Geometry: final body of the model. Coordinates: model frame, mm. A direction names the side the tool comes from. Give positions to 0.01 mm unless a question says otherwise; leave off trailing zeros. Loops run counter-clockwise (first coordinate to the right, second up) from the corner with the lowest first, then second, coordinate; pieces in that order, holes last.
from build123d import *

# Parameters (mm, degrees)
ESQUISSE1_W             = 80
ESQUISSE1_H             = 35
BOSS_EXTRU_1_DEPTH      = 5
ESQUISSE2_R             = 1.5
ESQUISSE2_R_2           = 1.3
ENL_V_MAT_EXTRU_1_DEPTH = 88.464278423
ESQUISSE4_R             = 2.5
ENL_V_MAT_EXTRU_2_DEPTH = 3
CONG_1_R                = 3


with BuildPart() as part:
    # Esquisse1 → Boss.-Extru.1 (new body)
    with BuildSketch(Plane(origin=(0, 0, 0), x_dir=(1, 0, 0), z_dir=(0, 1, 0))):
        with Locations((40, 17.5)):
            Rectangle(ESQUISSE1_W, ESQUISSE1_H)
    extrude(amount=BOSS_EXTRU_1_DEPTH)

    # Esquisse2 → Enlèv. mat.-Extru.1 (cut, through all)
    with BuildSketch(Plane(origin=(0, 5, 0), x_dir=(1, 0, 0), z_dir=(0, 1, 0))):
        with Locations(Location((5.5, 30, 0), (0, 0, 270))):
            Circle(ESQUISSE2_R)
        with Locations(Location((74.5, 30, 0), (0, 0, 270))):
            Circle(ESQUISSE2_R)
        with Locations(Location((29.270489512, 17.5, 0), (0, 0, 270))):
            Circle(ESQUISSE2_R_2)
        with Locations(Location((54.270489512, 17.5, 0), (0, 0, 270))):
            Circle(ESQUISSE2_R_2)
        with Locations(Location((74.5, 5, 0), (0, 0, 270))):
            Circle(ESQUISSE2_R)
        with Locations(Location((5.5, 5, 0), (0, 0, 270))):
            Circle(ESQUISSE2_R)
        with BuildLine():
            Line((71.602501664, 24.310381411), (71.602501664, 10.689618589))
            ThreePointArc((71.602501664, 10.689618589), (67.680448662, 6.767565587), (63.75839566, 10.689618589))
            Line((63.75839566, 10.689618589), (63.75839566, 24.310381411))
            ThreePointArc((63.75839566, 24.310381411), (67.680448662, 28.232434413), (71.602501664, 24.310381411))
        make_face()
        with BuildLine():
            Line((44.815714141, 24.310381411), (44.815714141, 10.689618589))
            ThreePointArc((44.815714141, 10.689618589), (40.893661139, 6.767565587), (36.971608137, 10.689618589))
            Line((36.971608137, 10.689618589), (36.971608137, 24.310381411))
            ThreePointArc((36.971608137, 24.310381411), (40.893661139, 28.232434413), (44.815714141, 24.310381411))
        make_face()
        with BuildLine():
            Line((20.115125023, 24.310381411), (20.115125023, 10.689618589))
            ThreePointArc((20.115125023, 10.689618589), (16.193072021, 6.767565587), (12.271019019, 10.689618589))
            Line((12.271019019, 10.689618589), (12.271019019, 24.310381411))
            ThreePointArc((12.271019019, 24.310381411), (16.193072021, 28.232434413), (20.115125023, 24.310381411))
        make_face()
    extrude(amount=-ENL_V_MAT_EXTRU_1_DEPTH, mode=Mode.SUBTRACT)

    # Esquisse4 → Enlèv. mat.-Extru.2 (cut)
    with BuildSketch(Plane(origin=(0, 5, 0), x_dir=(1, 0, 0), z_dir=(0, 1, 0))):
        with Locations(Location((29.270489512, 17.5, 0), (0, 0, 270))):
            Circle(ESQUISSE4_R)
        with Locations(Location((54.270489512, 17.5, 0), (0, 0, 270))):
            Circle(ESQUISSE4_R)
    extrude(amount=-ENL_V_MAT_EXTRU_2_DEPTH, mode=Mode.SUBTRACT)

    # Congé1
    cong_1_edges = [part.edges().sort_by_distance(p)[0] for p in [
        (0, 2.5, -35),
        (80, 2.5, -35),
        (80, 2.5, 0),
        (0, 2.5, 0),
    ]]
    fillet(cong_1_edges, radius=CONG_1_R)


solid = part.part
Item 1: Ray query, probe 1 along Z at (x, y) = (74.5, 3.6); probe 2 along X at (y, z) = (1.1, -5); probe 3 along X at (y, z) = (4.4, -22.5). Return the intervals inside material, ascending.
Values follow:
probe 1: z = -35 to -31.5, -28.5 to -6.5, -3.5 to 0
probe 2: x = 0 to 4, 7 to 73, 76 to 80
probe 3: x = 0 to 12.27, 20.12 to 36.97, 44.82 to 63.76, 71.6 to 80
Item 2: Section query C-C on z = -30. Return loops of the section in (x, y).
Values follow:
outline: (0, 0) - (4, 0) - (4, 5) - (0, 5) - close; (7, 0) - (73, 0) - (73, 5) - (7, 5) - close; (76, 0) - (80, 0) - (80, 5) - (76, 5) - close
Item 3: Draft query along X for faces 1 (the face through (79.1, 2.54, -34.14)), 2 (the face through (67.59, 2.54, -28.23)), 3 (the face through (39, 2, 0)), 4 (the face through (0.86, 2.54, -0.9)). Return one class per face: +X half, -X half, draft (parallel to the pull), parting line (faces both ways), or undercut.
Values follow:
face 1: +X half
face 2: undercut
face 3: draft
face 4: -X half
Item 4: Section query B-B on x = 5.5. Return loops of the section in (y, z), plus the area to 3 significant figures.
Values follow:
outline: (0, -35) - (5, -35) - (5, -31.5) - (0, -31.5) - close; (0, -28.5) - (5, -28.5) - (5, -6.5) - (0, -6.5) - close; (0, -3.5) - (5, -3.5) - (5, 0) - (0, 0) - close
area: 145 mm2
Item 5: Pin query (flat end, axial travel): pin 1 (3 mm diameter, centred on x = 29.27, z = -17.5, fed in from +Y). Return the tip coordinate at first contact, or that it passes through.
Values follow:
pin 1: stops at y = 2
Item 6: Section query A-A on z = -17.5. Give the number of separate pieces and of enclosed holes in the cut face, plus the area to 3 significant figures.
Values follow:
separate pieces: 6
enclosed holes: 0
area: 242 mm2
Item 7: Set-up query: faces 5 (the face through (12.271, 3, -17)), 6 (the face through (29.38, 3.521, -19.998)), 7 (the face through (31, 5, -14)). Return all of +Z, -Z, +X, -X, +Y, -Y with unobstructed straight access to the full face (end or side cutting, diameter ignored); none if empty.
Values follow:
face 5: +Y, -Y
face 6: +Y
face 7: +Z, -Z, +X, -X, +Y
